Input: part model. Units: mm. Frame: model coordinates. Face numbers are marked on the shaded views. A direction names the side the tool comes from. Round coordinates to 2 decimals unless told otherwise and drop trailing zeros. Loops run counter-clockwise (first coordinate to the right, second up) from the corner with the lowest first, then second, coordinate; pieces in that order, holes last. Notation, with made-up numbers: (35.25, -19.5) -> (65.25, -19.5) arc R27 ccw to (65.25, 7.5) -> close; hole circle Ø8 at (5, 2). An arc over 180 degrees is marked (long way). Answer as a JSON object with one key per item and string values. Group by question number.
Item 1: Section query D-D on z = -18.5. Return loops of the section in (x, y) (1 decimal), and give its area (3 significant figures).
Item 2: Section query C-C on y = 0. Count the separate pieces of the cut face and the enclosed holes in it, and give its area (3 significant figures).
Item 3: Section query B-B on x = 0. Return loops of the section in (y, z) (1 decimal).
Item 4: Section query A-A on z = 6.5. Return loops of the section in (x, y) (1 decimal).
Item 5: Pin query (flat end, axial travel): pin 1 (10 mm diameter, centred on x = 0, y = -12.7, fed in from +Z); pin 2 (12 mm diameter, centred on x = -2, y = 14, fed in from +Z) (3 decimals); pin 3 (2.5 mm diameter, centred on y = 0, z = -40.96, fed in from +X); pin 4 (1 mm diameter, centred on x = 4.5, z = -16, fed in from -Y). Return the tip coordinate at first contact, or that it passes through.
Item 6: Draft query along X for the marked faces 1, 2 and 3. Return one class per face: released by +X, released by -X, zero draft, split by the parting line, or undercut.
Item 7: Material intervals for line 1 (Y direction, x = 0, z = 7); line 2 (Z direction, x = -0.5, y = 0) (1 decimal); line 3 (Y direction, x = 5, z = 4.5), sorted ascending. Write a range as [from, to].
Item 8: Set-up query: the marked faces 4 and 5. Return all of +Z, -Z, +X, -X, +Y, -Y with unobstructed straight access to the full face (end or side cutting, diameter ignored); none if empty.
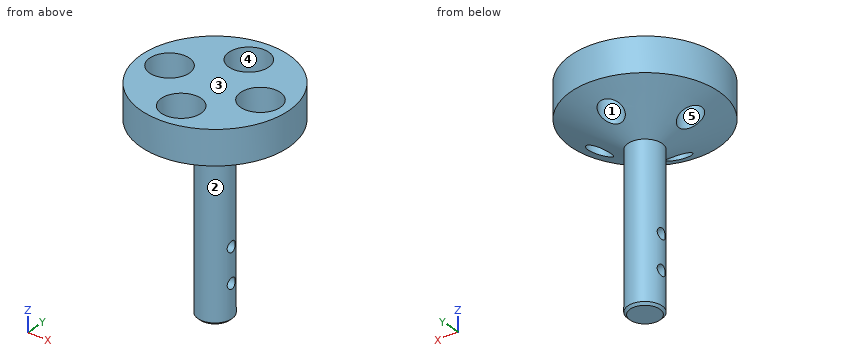
from build123d import *

# Parameters (mm, degrees)
SKETCH1_R               = 20.6375
BOSS_EXTRUDE1_DEPTH     = 9.525
SKETCH3_R               = 5.5626
CUT_EXTRUDE1_DEPTH      = 6.604
CIRPATTERN1_COUNT       = 4
SKETCH10_R              = 4.7625
BOSS_EXTRUDE3_DEPTH     = 50.8
CUT_EXTRUDE3_DEPTH      = 59.587138627
CUT_EXTRUDE3_DEPTH_BACK = 59.587138627
SKETCH11_R              = 1.5
SKETCH13_R              = 3.175
CUT_EXTRUDE4_DEPTH      = 62.13721178
CIRPATTERN2_COUNT       = 4
CHAMFER1_SIZE           = 0.635


with BuildPart() as part:
    # Sketch1 → Boss-Extrude1 (new body)
    with BuildSketch(Plane.XY):
        with Locations(Location((0, 0, 0), (0, 0, 180))):
            Circle(SKETCH1_R)
    extrude(amount=BOSS_EXTRUDE1_DEPTH)

    # Sketch3 → Cut-Extrude1 (cut)
    with BuildSketch(Plane.XY.offset(9.525)):
        with Locations((0, 12.7)):
            Circle(SKETCH3_R)
    cut_extrude1 = extrude(amount=-CUT_EXTRUDE1_DEPTH, mode=Mode.SUBTRACT)

    # CirPattern1: Cut-Extrude1 ×4 about axis
    cirpattern1_axis = Axis((0, 0, 0), (0, 0, 1))
    for i in range(1, CIRPATTERN1_COUNT):
        add(cut_extrude1.rotate(cirpattern1_axis, i * 360 / CIRPATTERN1_COUNT), mode=Mode.SUBTRACT)

    # Sketch10 → Boss-Extrude3 (add)
    with BuildSketch(Plane(origin=(0, 0, 0), x_dir=(-1, 0, 0), z_dir=(0, 0, -1))):
        Circle(SKETCH10_R)
    extrude(amount=BOSS_EXTRUDE3_DEPTH)

    # Sketch11 → Cut-Extrude3 (cut, two sides: drawn at the far end of the back side and taken through both)
    with BuildSketch(Plane(origin=(0, 0, 0), x_dir=(0, 0, -1), z_dir=(1, 0, 0)).offset(-CUT_EXTRUDE3_DEPTH_BACK)):
        with Locations((31.4325, 0)):
            Circle(SKETCH11_R)
        with Locations((40.9575, 0)):
            Circle(SKETCH11_R)
    extrude(amount=CUT_EXTRUDE3_DEPTH + CUT_EXTRUDE3_DEPTH_BACK, mode=Mode.SUBTRACT)

    # Sketch12 → Revolve1 (revolve)
    with BuildSketch(Plane(origin=(0, 0, 0), x_dir=(1, 0, 0), z_dir=(0, 1, 0)), mode=Mode.PRIVATE) as revolve1_sk:
        Polygon((-20.6375, 0), (-4.7625, 7.9375), (-4.7625, 0), align=None)
    revolve(revolve1_sk.sketch.rotate(Axis((0, 0, 0), (0, 0, -1)), 180), axis=Axis((0, 0, 0), (0, 0, -1)))

    # Sketch13 → Cut-Extrude4 (cut, through all)
    with BuildSketch(Plane.XY.offset(2.921)):
        with Locations((-12.7, 0)):
            Circle(SKETCH13_R)
    cut_extrude4 = extrude(amount=-CUT_EXTRUDE4_DEPTH, mode=Mode.SUBTRACT)

    # CirPattern2: Cut-Extrude4 ×4 about axis
    cirpattern2_axis = Axis((0, 0, 0), (0, 0, 1))
    for i in range(1, CIRPATTERN2_COUNT):
        add(cut_extrude4.rotate(cirpattern2_axis, i * 360 / CIRPATTERN2_COUNT), mode=Mode.SUBTRACT)

    # Chamfer1
    chamfer1_edges = [part.edges().sort_by_distance(p)[0] for p in [
        (4.7625, 0, -50.8),
    ]]
    chamfer(chamfer1_edges, length=CHAMFER1_SIZE)


solid = part.part
Solved:
{
 "1": {"outline": "circle Ø9.5 at (0, 0)", "area": "71.3 mm²"},
 "2": {"separate pieces": "5", "enclosed holes": "0", "area": "711 mm²"},
 "3": {"outline": "(-20.6, 0) -> (-15.9, -2.4) -> (-15.9, 2.9) -> (-18.3, 2.9) -> (-18.3, 9.5) -> (-20.6, 9.5) -> close; (-9.5, -5.6) -> (-4.8, -7.9) -> (-4.8, -50.2) -> (-4.1, -50.8) -> (4.1, -50.8) -> (4.8, -50.2) -> (4.8, -7.9) -> (9.5, -5.6) -> (9.5, 2.9) -> (7.1, 2.9) -> (7.1, 9.5) -> (-7.1, 9.5) -> (-7.1, 2.9) -> (-9.5, 2.9) -> close; (15.9, -2.4) -> (20.6, 0) -> (20.6, 9.5) -> (18.3, 9.5) -> (18.3, 2.9) -> (15.9, 2.9) -> close; hole circle Ø3 at (0, -41); hole circle Ø3 at (0, -31.4)"},
 "4": {"outline": "circle Ø41.3 at (0, 0); hole circle Ø11.1 at (-12.7, 0); hole circle Ø11.1 at (0, -12.7); hole circle Ø11.1 at (0, 12.7); hole circle Ø11.1 at (12.7, 0)"},
 "5": {"pin 1": "z = 2.92", "pin 2": "z = 9.525", "pin 3": "through", "pin 4": "y = -2.58"},
 "6": {"face 1": "undercut", "face 2": "split by the parting line", "face 3": "zero draft"},
 "7": {"line 1": "[-20.64, -18.26], [-7.14, 7.14], [18.26, 20.64]", "line 2": "[-50.8, -42.5], [-39.5, -32.9], [-29.9, 9.5]", "line 3": "[-20.02, -15.14], [-10.26, 10.26], [15.14, 20.02]"},
 "8": {"face 4": "+Z", "face 5": "+Z, -Z"}
}
